Geometry check sheet. Reference: the model listing, model coordinates, mm. A direction names the side the tool comes from. Give positions to 0.01 mm unless a question says otherwise; leave off trailing zeros. Loops run counter-clockwise (first coordinate to the right, second up) from the corner with the lowest first, then second, coordinate; pieces in that order, holes last. Notation, with made-up numbers: (7.5, -24) - (43.5, -24) arc R23 cw to (43.5, 9) - close; hole circle Ø6 at (-25, 75). An arc over 180 degrees is marked (long way). Write item = value, one per line. Start each with the question number.
from build123d import *

# Parameters (mm, degrees)
SKETCH1_R           = 75
BOSS_EXTRUDE1_DEPTH = 10
SKETCH2_R           = 50
SKETCH2_R_2         = 25
BOSS_EXTRUDE2_DEPTH = 50
BOSS_EXTRUDE4_DEPTH = 50
CIRPATTERN2_COUNT   = 6
SKETCH5_R           = 2.5
CUT_EXTRUDE5_DEPTH  = 5
CIRPATTERN3_COUNT   = 6


with BuildPart() as part:
    # Sketch1 → Boss-Extrude1 (new body)
    with BuildSketch(Plane(origin=(0, 0, 0), x_dir=(1, 0, 0), z_dir=(0, 1, 0))):
        with Locations(Location((0, 0, 0), (0, 0, 270))):
            Circle(SKETCH1_R)
    extrude(amount=BOSS_EXTRUDE1_DEPTH)

    # Sketch2 → Boss-Extrude2 (add)
    with BuildSketch(Plane(origin=(0, 10, 0), x_dir=(1, 0, 0), z_dir=(0, 1, 0))):
        with Locations(Location((0, 0, 0), (0, 0, 270))):
            Circle(SKETCH2_R)
        with Locations(Location((0, 0, 0), (0, 0, 270))):
            Circle(SKETCH2_R_2, mode=Mode.SUBTRACT)
    extrude(amount=BOSS_EXTRUDE2_DEPTH)

    # Sketch3 → Boss-Extrude4 (add)
    with BuildSketch(Plane(origin=(0, 10, 0), x_dir=(1, 0, 0), z_dir=(0, 1, 0))):
        with BuildLine():
            ThreePointArc((5, 74.833147735), (0, 75), (-5, 74.833147735))
            Line((-5, 74.833147735), (-5, 49.749371855))
            ThreePointArc((-5, 49.749371855), (0, 50), (5, 49.749371855))
            Line((5, 49.749371855), (5, 74.833147735))
        make_face()
        with BuildLine():
            Line((5, -74.833147735), (5, -49.749371855))
            ThreePointArc((5, -49.749371855), (0, -50), (-5, -49.749371855))
            Line((-5, -49.749371855), (-5, -74.833147735))
            ThreePointArc((-5, -74.833147735), (0, -75), (5, -74.833147735))
        make_face()
    boss_extrude4 = extrude(amount=BOSS_EXTRUDE4_DEPTH)

    # CirPattern2: Boss-Extrude4 ×6 about axis
    cirpattern2_axis = Axis((0, 0, 0), (0, 1, 0))
    for i in range(1, CIRPATTERN2_COUNT):
        add(boss_extrude4.rotate(cirpattern2_axis, i * 360 / CIRPATTERN2_COUNT))

    # Sketch5 → Cut-Extrude5 (cut)
    with BuildSketch(Plane(origin=(0, 10, 0), x_dir=(1, 0, 0), z_dir=(0, 1, 0))):
        with Locations(Location((-62.5, 0, 0), (0, 0, 270))):
            Circle(SKETCH5_R)
    cut_extrude5 = extrude(amount=-CUT_EXTRUDE5_DEPTH, mode=Mode.SUBTRACT)

    # CirPattern3: Cut-Extrude5 ×6 about axis
    cirpattern3_axis = Axis((0, 0, 0), (0, 1, 0))
    for i in range(1, CIRPATTERN3_COUNT):
        add(cut_extrude5.rotate(cirpattern3_axis, i * 360 / CIRPATTERN3_COUNT), mode=Mode.SUBTRACT)


solid = part.part
1) Cross-section at A-A on y = 51. Enter the section's corners in (x, z), and give its area (3 significant figures).
2) Gauge pin test, flat ends, axial feed: P1, Ø8, axis at x = -62.5, z = 0, coming from the -Y side; P2, Ø2.5, axis at x = -31.5, z = 54.5, coming from the +Y side; P3, Ø10, axis at x = -42.5, y = 20, coming from the -Z side; P4, Ø13.5, axis at x = 46.5, z = 47.5, coming from the +Y side. Record the tip position at first contact, or that the pin passes through.
3) Material ranges on line 1 along X through (y, z) = (8, 0); line 2 along X through (y, z) = (40, 0); line 3 along Y through (x, z) = (-64, -13.5), recorded low to high.
4) Cross-section at B-B on z = 0. Enter the section's corners in (x, y).
5) Tool access check on faces 1 (the face through (-56.294, 34.65, 26.728)), 2 (the face through (-33, 10, 52)), 3 (the face through (25.26, 34.65, -43.15)), 4 (the face through (56.294, 34.65, -26.728)), 5 (the face through (31, 5, 54)). Record the directions out of +Z, -Z, +X, -X, +Y, -Y that give a thin tool (end or side, any length) a straight path to the whole face; none if there is none.
6) Cross-section at D-D on x = -31.25. Enter the section's corners in (y, z).
7) Cross-section at C-C on x = 0. Enter the section's corners in (y, z), and give its area (3 significant figures).
Checked values:
q1.outline = (-67.31, -33.09) arc R75 ccw to (-62.31, -41.75) - (-40.58, -29.2) arc R50 ccw to (-5, -49.75) - (-5, -74.83) arc R75 ccw to (5, -74.83) - (5, -49.75) arc R50 ccw to (40.58, -29.2) - (62.31, -41.75) arc R75 ccw to (67.31, -33.09) - (45.58, -20.54) arc R50 ccw to (45.58, 20.54) - (67.31, 33.09) arc R75 ccw to (62.31, 41.75) - (40.58, 29.2) arc R50 ccw to (5, 49.75) - (5, 74.83) arc R75 ccw to (-5, 74.83) - (-5, 49.75) arc R50 ccw to (-40.58, 29.2) - (-62.31, 41.75) arc R75 ccw to (-67.31, 33.09) - (-45.58, 20.54) arc R50 ccw to (-45.58, -20.54) - close; hole circle Ø50 at (0, 0)
q1.area = 7,390 mm²
q2.P1 = 0
q2.P2 = 5
q2.P3 = -33.2
q2.P4 = 10
q3.line_1 = -75 to -65, -60 to 60, 65 to 75
q3.line_2 = -50 to -25, 25 to 50
q3.line_3 = 0 to 10
q4.outline = (-75, 0) - (75, 0) - (75, 10) - (65, 10) - (65, 5) - (60, 5) - (60, 10) - (50, 10) - (50, 60) - (25, 60) - (25, 10) - (-25, 10) - (-25, 60) - (-50, 60) - (-50, 10) - (-60, 10) - (-60, 5) - (-65, 5) - (-65, 10) - (-75, 10) - close
q5.face_1 = -X, +Y
q5.face_2 = +Z, +Y
q5.face_3 = -Z, +Y
q5.face_4 = +X, +Y
q5.face_5 = +Y
q6.outline = (0, -68.18) - (10, -68.18) - (10, -56.63) - (5, -56.63) - (5, -51.63) - (10, -51.63) - (10, -39.03) - (60, -39.03) - (60, 39.03) - (10, 39.03) - (10, 51.63) - (5, 51.63) - (5, 56.63) - (10, 56.63) - (10, 68.18) - (0, 68.18) - close
q7.outline = (0, -75) - (60, -75) - (60, -25) - (10, -25) - (10, 25) - (60, 25) - (60, 75) - (0, 75) - close
q7.area = 6,500 mm²
